```python
from build123d import *

# Parameters (mm, degrees)
SKETCH1_R                                       = 0.5
BOSS_EXTRUDE1_DEPTH                             = 18
FILLET2_R                                       = 1
CSK_FOR_M3_FLAT_HEAD_MACHINE_SCREW2_D           = 3.4
CSK_FOR_M3_FLAT_HEAD_MACHINE_SCREW2_CSINK_D     = 6.3
CSK_FOR_M3_FLAT_HEAD_MACHINE_SCREW2_CSINK_ANGLE = 90


with BuildPart() as part:
    # Sketch1 → Boss-Extrude1 (new body)
    with BuildSketch(Plane(origin=(0, 0, 0), x_dir=(1, 0, 0), z_dir=(0, 1, 0))):
        with BuildLine():
            Line((-2.5, -17.994062369), (-2.5, 0))
            ThreePointArc((-2.5, 0), (0, 2.5), (2.5, 0))
            Line((2.5, 0), (2.5, -18.006040941))
            Line((2.5, -18.006040941), (-2.5, -17.994062369))
        make_face()
        with Locations(Location((0, 0, 0), (0, 0, 270))):
            Circle(SKETCH1_R, mode=Mode.SUBTRACT)
    extrude(amount=BOSS_EXTRUDE1_DEPTH)

    # Fillet2
    fillet2_edges = [part.edges().sort_by_distance(p)[0] for p in [
        (0, 18, 18.000051655),
        (0, 0, 18.000051655),
    ]]
    fillet(fillet2_edges, radius=FILLET2_R)

    # CSK for M3 Flat Head Machine Screw2 (through all)
    with Locations(Plane.ZY.offset(2.5)):
        with Locations((5.7, 9), (13, 9)):
            CounterSinkHole(CSK_FOR_M3_FLAT_HEAD_MACHINE_SCREW2_D / 2, CSK_FOR_M3_FLAT_HEAD_MACHINE_SCREW2_CSINK_D / 2, counter_sink_angle=CSK_FOR_M3_FLAT_HEAD_MACHINE_SCREW2_CSINK_ANGLE)


solid = part.part
```
Check sheet for the modelled part. Datum: model origin and axes. Units: mm. Give positions to 0.01 mm unless a question says otherwise; leave off trailing zeros. Order: outer loops, then holes, each group sorted by start corner. A loop starts at its lowest first (then second) coordinate and runs counter-clockwise, first axis right, second up. Notation, with made-up numbers: (3, -8) -> (37, -8) arc R18 cw to (37, 17) -> close; hole circle Ø10 at (77, 70.5). An arc over 180 degrees is marked (long way). Use CSV: the item, a comma, the result in double quotes. Start each with the question number.
1) Sectioned sample at A-A, the plane z = 5.7. Record the boundary of the cut face in (x, y).
2) Mould release check, pull along Y, two halves, no side actions. Record for faces 1 (the face through (2.5, 9, 9)), 2 (the face through (0, 0, 7)), 3 (the face through (0.7, 7.5, 4.9)): released by +Y, released by -Y, zero draft, split by the parting line, or undercut.
3) Material ranges on line 1 (Y direction, x = 0.1, z = 13); line 2 (X direction, y = 12, z = 0); line 3 (Z direction, x = -0.1, y = 9), recorded low to high. Write a range as from..to.
4) Sectioned sample at C-C, the plane y = 12.75. Record the boundary of the cut face in (x, z), plus the area to 3 significant figures.
5) Go/stop test with flat-tipped pins: P1, Ø2, axis at y = 9, z = 5.7, coming from the +X side; P2, Ø6, axis at y = 9, z = 3.5, coming from the -X side; P3, Ø1, axis at x = -0.5, y = 3.5, coming from the +Z side; P4, Ø3, axis at y = 9, z = 14, coming from the -X side. Record where each tip stops, or that it passes through.
6) Sectioned sample at D-D, the plane x = 0. Give the number of separate pieces and of enclosed holes in the cut face, plus the area to 3 significant figures.
7) Sectioned sample at B-B, the plane y = 9. Record the boundary of the cut face in (x, z).
Recorded:
1,outline,"(-2.5, 0) -> (2.5, 0) -> (2.5, 7.3) -> (-1.05, 7.3) -> (-2.5, 5.85) -> close; (-2.5, 12.15) -> (-1.05, 10.7) -> (2.5, 10.7) -> (2.5, 18) -> (-2.5, 18) -> close"
2,face 1,"zero draft"
2,face 2,"released by -Y"
2,face 3,"undercut"
3,line 1,"0..7.3, 10.7..18"
3,line 2,"-2.5..-0.5, 0.5..2.5"
3,line 3,"-2.5..-0.49, 0.49..4, 7.4..11.3, 14.7..18"
4,outline,"(-2.5, 0) arc R2.5 ccw to (2.5, 0) -> (2.5, 18.01) -> (-2.5, 17.99) -> close; hole circle Ø1 at (0, 0)"
4,area,"99.0 mm2"
5,P1,"through"
5,P2,"x = -2.5"
5,P3,"z = 18"
5,P4,"x = -1.85"
6,separate pieces,"2"
6,enclosed holes,"2"
6,area,"332 mm2"
7,outline,"(-2.5, 0) arc R2.5 ccw to (2.5, 0) -> (2.5, 4) -> (-1.05, 4) -> (-2.5, 2.55) -> close; (-2.5, 8.85) -> (-1.05, 7.4) -> (2.5, 7.4) -> (2.5, 11.3) -> (-1.05, 11.3) -> (-2.5, 9.85) -> close; (-2.5, 16.15) -> (-1.05, 14.7) -> (2.5, 14.7) -> (2.5, 18.01) -> (-2.5, 17.99) -> close; hole circle Ø1 at (0, 0)"
